The listing builds one solid part. Answer for the finished solid, in the listing's coordinates (mm). Face numbers are marked on the shaded views. Coordinates: 2 decimals unless noted, no trailing zeros. Order: outer loops, then holes, each group sorted by start corner. A loop starts at its lowest first (then second) coordinate and runs counter-clockwise, first axis right, second up.
from build123d import *

# Parameters (mm, degrees)
SKETCH2_R               = 43.815
SKETCH2_R_2             = 40
BASE_CYLINDER_DEPTH     = 381
SKETCH3_R               = 56.35625
SKETCH3_R_2             = 40
AFT_FLANGE_DEPTH        = 9.525
SKETCH6_R               = 46.9011
SKETCH6_R_2             = 44.2849
AFT_O_RING_DEPTH        = 1.9812
SKETCH33_R              = 45.72
SKETCH33_R_2            = 43.815
CRITICALBOSS_DEPTH      = 22.225
FILLET1_R               = 2.54
BOLT_CIRCLE_D           = 2.2606
BOLT_CIRCLE_DEPTH       = 381
HOLE1_D                 = 2.38125
HOLE1_DEPTH             = 381
HOLE1_CBORE_D           = 4.7625
HOLE1_CBORE_DEPTH       = 4.7625
F_3_8_24_TAPPED_HOLE1_D = 8.4328
FILLET2_R               = 2.54


with BuildPart() as part:
    # Sketch2 → Base Cylinder (new body)
    with BuildSketch(Plane(origin=(0, 0, 0), x_dir=(1, 0, 0), z_dir=(0, 1, 0))):
        with Locations(Location((0, 0, 0), (0, 0, 270))):
            Circle(SKETCH2_R)
        with Locations(Location((0, 0, 0), (0, 0, 270))):
            Circle(SKETCH2_R_2, mode=Mode.SUBTRACT)
    extrude(amount=BASE_CYLINDER_DEPTH)

    # Sketch3 → Aft Flange (add)
    with BuildSketch(Plane.XZ):
        with Locations(Location((0, 0, 0), (0, 0, 270))):
            Circle(SKETCH3_R)
        with Locations(Location((0, 0, 0), (0, 0, 90))):
            Circle(SKETCH3_R_2, mode=Mode.SUBTRACT)
    aft_flange = extrude(amount=-AFT_FLANGE_DEPTH)

    # Sketch6 → Aft O-Ring (cut)
    with BuildSketch(Plane.XZ):
        with Locations(Location((0, 0, 0), (0, 0, 270))):
            Circle(SKETCH6_R)
        with Locations(Location((0, 0, 0), (0, 0, 270))):
            Circle(SKETCH6_R_2, mode=Mode.SUBTRACT)
    aft_o_ring = extrude(amount=-AFT_O_RING_DEPTH, mode=Mode.SUBTRACT)

    # Sketch33 → CriticalBoss (add)
    with BuildSketch(Plane(origin=(0, 9.525, 0), x_dir=(1, 0, 0), z_dir=(0, 1, 0))):
        with Locations(Location((0, 0, 0), (0, 0, 90))):
            Circle(SKETCH33_R)
        with Locations(Location((0, 0, 0), (0, 0, 270))):
            Circle(SKETCH33_R_2, mode=Mode.SUBTRACT)
    extrude(amount=CRITICALBOSS_DEPTH)

    # Fillet1
    # the kernel refuses this fillet: 2.54 mm, written as the material it adds along each edge
    with BuildSketch(Plane(origin=(0, 9.525, 0), x_dir=(0, 0, -1), z_dir=(1, 0, 0))) as fillet1_piece_1:
        with BuildLine():
            CenterArc((45.72 + FILLET1_R, FILLET1_R), FILLET1_R, 180, 90)
            Line((45.72, FILLET1_R), (45.72 - FILLET1_R * 0.02, FILLET1_R))
            Line((45.72 - FILLET1_R * 0.02, FILLET1_R), (45.72 - FILLET1_R * 0.02, -FILLET1_R * 0.02))
            Line((45.72 - FILLET1_R * 0.02, -FILLET1_R * 0.02), (45.72 + FILLET1_R, -FILLET1_R * 0.02))
            Line((45.72 + FILLET1_R, -FILLET1_R * 0.02), (45.72 + FILLET1_R, 0))
        make_face()
    revolve(axis=Axis((0, 9.525, 0), (0, 1, 0)))
    with BuildSketch(Plane(origin=(0, 31.75, 0), x_dir=(0, 0, 1), z_dir=(-1, 0, 0))) as fillet1_piece_2:
        with BuildLine():
            CenterArc((46.355, 2.459344425), FILLET1_R, 180, 75.522487814)
            Line((43.815, 2.459344425), (43.7642, 2.459344425))
            Line((43.7642, 2.459344425), (43.7642, 0))
            Line((43.7642, 0), (43.815, -0.0508))
            ThreePointArc((43.815, -0.0508), (44.7675, -0.0508), (45.7073, -0.049186888))
            Line((45.7073, -0.049186888), (45.72, 0))
        make_face()
    revolve(axis=Axis((0, 31.75, 0), (0, 1, 0)))

    # Bolt Circle
    with Locations(Plane(origin=(0, 0, 0), x_dir=(-1, 0, 0), z_dir=(0, -1, 0))):
        with Locations((-25.81275, -44.708994483), (-44.708994483, -25.81275), (-51.6255, 0), (-44.708994483, 25.81275), (-25.81275, 44.708994483), (0, 51.6255), (25.81275, 44.708994483), (44.708994483, 25.81275), (51.6255, 0), (44.708994483, -25.81275), (25.81275, -44.708994483), (0, -51.6255)):
            bolt_circle = Hole(BOLT_CIRCLE_D / 2, depth=BOLT_CIRCLE_DEPTH)

    # Hole1
    with Locations(Plane(origin=(0, 0, 0), x_dir=(-1, 0, 0), z_dir=(0, -1, 0))):
        with Locations((49.866403745, 13.361662613), (-49.866403745, -13.361662613)):
            hole1 = CounterBoreHole(HOLE1_D / 2, HOLE1_CBORE_D / 2, HOLE1_CBORE_DEPTH, depth=HOLE1_DEPTH)

    # Sketch44 → 1/8 NPT Tapped ThermocoupleHole (revolve, cut)
    with BuildSketch(Plane(origin=(0, 22.225, -45.72), x_dir=(0, 1, 0), z_dir=(1, 0, 0))):
        Polygon((0, 0), (0, 14.217468714), (4.2164, 11.684), (4.2164, 6.858), (4.936181096, 6.858), (5.1415188, 0), align=None)
    revolve(axis=Axis((0, 22.225, -52.07), (0, 0, 1)), mode=Mode.SUBTRACT)

    # 3/8-24 Tapped Hole1 (through all)
    with Locations(Plane.XY.offset(45.72)):
        with Locations((0, 22.225)):
            Hole(F_3_8_24_TAPPED_HOLE1_D / 2)

    # Mirror1: Aft Flange, Aft O-Ring, Bolt Circle, Hole1 across plane
    add(aft_flange.mirror(Plane.ZX.offset(190.5)))
    add(aft_o_ring.mirror(Plane.ZX.offset(190.5)), mode=Mode.SUBTRACT)
    add(bolt_circle.mirror(Plane.ZX.offset(190.5)), mode=Mode.SUBTRACT)
    add(hole1.mirror(Plane.ZX.offset(190.5)), mode=Mode.SUBTRACT)

    # Fillet2
    fillet2_edges = [part.edges().sort_by_distance(p)[0] for p in [
        (0, 371.475, -43.815),
    ]]
    fillet(fillet2_edges, radius=FILLET2_R)


solid = part.part
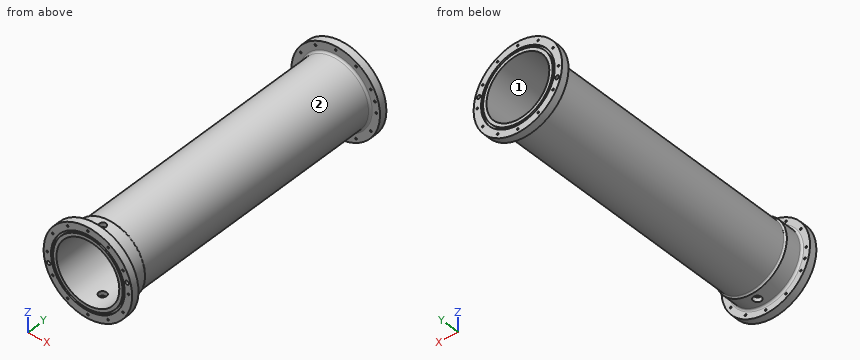
(1) Given pin 1 Ø4 at (x, y) = (-42.5, 266) entering from -Z; pin 2 Ø3 at (x, y) = (-26, 255.5) entering from -Z (3 decimals); pin 3 Ø1 at (x, y) = (-40, 118.5) entering from +Z, each flat-ended and moving along its own axis, determine where each tip first touches the part or whether it passes through.
(2) Find section A-A on y = 47. Determine the outline of the cut face in (x, z) (3 decimals), then the cut area to 3 significant figures.
(3) The mould has two halves that part along X. Classify the marked faces 1 and 2: pulls with the +X half, pulls with the -X half, needs draft (parallel to the pull), parting line crosses it, or undercut.
(4) Find the intervals of material crossed by probe 1 along Y at (x, z) = (-30, 39) (3 decimals); probe 2 along Z at (x, y) = (5.5, 276); probe 3 along X at (y, z) = (277.5, -15.5), in increasing order.
Resolved:
1. pin 1: stops at z = -16.72
1. pin 2: stops at z = -36.325
1. pin 3: stops at z = 18.96
2. outline: circle Ø87.63 at (0, 0); hole circle Ø80 at (0, 0)
2. area: 1,000 mm2
3. face 1: undercut
3. face 2: parting line crosses it
4. probe 1: y = 0 to 9.525, 371.475 to 381
4. probe 2: z = -43.47 to -39.62, 39.62 to 43.47
4. probe 3: x = -40.98 to -36.87, 36.87 to 40.98
